from build123d import *

# Parameters (mm, degrees)
F0_W     = 38.419276
F0_H     = 18.38255
F4_DEPTH = 9.475427
F1_SIZE  = 5.08
F2_W     = 31.43239
F2_H     = 13.718766
F3_DEPTH = 3.943906


with BuildPart() as f4:
    # F0 (on Front) → F4 (new body)
    with BuildSketch(Plane.XZ):
        Rectangle(F0_W, F0_H)
    extrude(amount=F4_DEPTH)

    # F1
    f1_edges = [f4.edges().sort_by_distance(p)[0] for p in [
        (19.209638, -9.475427, 0),
        (0, -9.475427, 9.191275),
        (-19.209638, -9.475427, 0),
        (0, -9.475427, -9.191275),
    ]]
    chamfer(f1_edges, length=F1_SIZE)

    # F2 (on face) → F3 (cut)
    with BuildSketch(Plane(origin=(0, 0, 0), x_dir=(-1, 0, 0), z_dir=(0, 1, 0))):
        Rectangle(F2_W, F2_H)
    extrude(amount=-F3_DEPTH, mode=Mode.SUBTRACT)


solid = f4.part
Read the model definition and answer for the solid it produces. Units are mm, in the model's axes. A direction names the side the tool comes from. Give positions to 0.01 mm unless a question says otherwise; leave off trailing zeros. Loops run counter-clockwise (first coordinate to the right, second up) from the corner with the lowest first, then second, coordinate; pieces in that order, holes last. Notation, with made-up numbers: (69.5, 4) -> (112.5, 4) arc R11 ccw to (112.5, 9) -> close; hole circle Ø3 at (66.25, 56.5). An arc over 180 degrees is marked (long way). Answer as CSV lines item,"result".
Item 1: Determine the mould class of faces 1 (the face through (0, -9.475, 0)), 2 (the face through (-15.716, -2, 0)), 3 (the face through (-0.269, -6.971, 6.616)) for opening direction Z: +Z half, -Z half, draft (parallel to the pull), parting line (faces both ways), or undercut.
Returned:
face 1,"draft"
face 2,"undercut"
face 3,"+Z half"
Item 2: Find section D-D on y = -7.75. Give the vertices of the cut face in (x, z).
Returned:
outline,"(-15.86, -5.84) -> (15.86, -5.84) -> (15.86, 5.84) -> (-15.86, 5.84) -> close"
Item 3: Consider line 1 (Z direction, x = -10, y = -1.25); line 2 (X direction, y = -3.5, z = -4.25); line 3 (Y direction, x = -2.5, z = 2.25). Determine where each line is inside the solid, lowest interval first. Write a range as [from, to].
Returned:
line 1,"z = [-9.19, -6.86], [6.86, 9.19]"
line 2,"x = [-19.21, -15.72], [15.72, 19.21]"
line 3,"y = [-9.48, -3.94]"
Item 4: For faces 4 (the face through (19.21, -2, 0)), 5 (the face through (0, -2, -6.859)), determine the directions among +Z, -Z, +X, -X, +Y, -Y from which every point of the face is accessible in a straight line to the end or side of a thin tool.
Returned:
face 4,"+Z, -Z, +X, +Y, -Y"
face 5,"+Y"
Item 5: This flat-tipped pin is pushed along its axis until it touches: pin 1 (4 mm diameter, centred on x = 7, z = 1, fed in from +Y). Where does it stop, or does it pass through?
Returned:
pin 1,"stops at y = -3.94"
Item 6: Find section B-B on z = -2.25. Give the vertices of the cut face in (x, y).
Returned:
outline,"(-19.21, -4.4) -> (-14.13, -9.48) -> (14.13, -9.48) -> (19.21, -4.4) -> (19.21, 0) -> (15.72, 0) -> (15.72, -3.94) -> (-15.72, -3.94) -> (-15.72, 0) -> (-19.21, 0) -> close"
Item 7: Find section C-C on x = 8.5. Give the vertices of the cut face in (y, z).
Returned:
outline,"(-9.48, -4.11) -> (-4.4, -9.19) -> (0, -9.19) -> (0, -6.86) -> (-3.94, -6.86) -> (-3.94, 6.86) -> (0, 6.86) -> (0, 9.19) -> (-4.4, 9.19) -> (-9.48, 4.11) -> close"
Item 8: Find section A-A on y = -3.5. Give the vertices of the cut face in (x, z), plus the area to 3 significant figures.
Returned:
outline,"(-19.21, -9.19) -> (19.21, -9.19) -> (19.21, 9.19) -> (-19.21, 9.19) -> close; hole (-15.72, -6.86) -> (15.72, -6.86) -> (15.72, 6.86) -> (-15.72, 6.86) -> close"
area,"275 mm²"
